For this review, take the finished solid that the model builds, in its own axes (mm). A direction names the side the tool comes from. Give positions to 0.01 mm unless a question says otherwise; leave off trailing zeros. Order: outer loops, then holes, each group sorted by start corner. A loop starts at its lowest first (then second) coordinate and runs counter-clockwise, first axis right, second up. Notation, with made-up numbers: (-20.5, 86.5) - (9.5, 86.5) arc R21 ccw to (9.5, 92.5) - close; hole circle Ø11 at (75, 26). An arc over 180 degrees is marked (long way). Put each result on its own line as item: value. Start each with the question number.
```python
from build123d import *

# Parameters (mm, degrees)
SKETCH1_W           = 69.43077851
SKETCH1_H           = 69.43077851
BOSS_EXTRUDE2_DEPTH = 3
SKETCH6_R           = 1.5
SKETCH6_W           = 50.43077851
SKETCH6_H           = 15.826208999
CUT_EXTRUDE1_DEPTH  = 10
FILLET1_R           = 10
FILLET2_R           = 10
FILLET3_R           = 4.994579941


with BuildPart() as part:
    # Sketch1 → Boss-Extrude2 (new body)
    with BuildSketch(Plane.XY):
        Rectangle(SKETCH1_W, SKETCH1_H)
    extrude(amount=BOSS_EXTRUDE2_DEPTH)

    # Sketch6 → Cut-Extrude1 (cut)
    with BuildSketch(Plane.XY.offset(3)):
        with Locations((-29, 24.5)):
            Circle(SKETCH6_R)
        with Locations((-29, -24.5)):
            Circle(SKETCH6_R)
        with Locations((29, -24.5)):
            Circle(SKETCH6_R)
        with Locations((29, 24.5)):
            Circle(SKETCH6_R)
        with Locations((0, -26.802284756)):
            Rectangle(SKETCH6_W, SKETCH6_H)
    extrude(amount=-CUT_EXTRUDE1_DEPTH, mode=Mode.SUBTRACT)

    # Fillet1
    fillet1_edges = [part.edges().sort_by_distance(p)[0] for p in [
        (34.715389255, 34.715389255, 1.5),
    ]]
    fillet(fillet1_edges, radius=FILLET1_R)

    # Fillet2
    # the kernel refuses this fillet: 10 mm, written as the material it takes off along each edge
    with BuildSketch(Plane(origin=(34.715389255, -34.715389255, -24.968730444), x_dir=(0, 1, 0), z_dir=(0, 0, 1))) as fillet2_piece_1:
        with BuildLine():
            CenterArc((9.987492178, 10), FILLET2_R, 182.865983983, 87.134016017)
            Line((0, 9.5), (-0.199749844, 9.49))
            ThreePointArc((-0.199749844, 9.49), (-0.2, 4.75), (-0.2, 0))
            Line((-0.2, 0), (0, -0.2))
            Line((0, -0.2), (9.987492178, -0.2))
            Line((9.987492178, -0.2), (9.987492178, 0))
        make_face()
    extrude(amount=52.937460889, mode=Mode.SUBTRACT)
    with BuildSketch(Plane(origin=(-34.715389255, -34.715389255, -24.968730444), x_dir=(0, 1, 0), z_dir=(0, 0, 1))) as fillet2_piece_2:
        with BuildLine():
            CenterArc((9.987492178, -10), FILLET2_R, 90, 87.134016017)
            Line((0, -9.5), (-0.199749844, -9.49))
            ThreePointArc((-0.199749844, -9.49), (-0.2, -4.75), (-0.2, 0))
            Line((-0.2, 0), (0, 0.2))
            Line((0, 0.2), (9.987492178, 0.2))
            Line((9.987492178, 0.2), (9.987492178, 0))
        make_face()
    extrude(amount=52.937460889, mode=Mode.SUBTRACT)
    with BuildSketch(Plane(origin=(-34.715389255, 34.715389255, -25), x_dir=(1, 0, 0), z_dir=(0, 0, 1))) as fillet2_piece_3:
        with BuildLine():
            CenterArc((FILLET2_R, -FILLET2_R), FILLET2_R, 90, 90)
            Line((0, -FILLET2_R), (-FILLET2_R * 0.02, -FILLET2_R))
            Line((-FILLET2_R * 0.02, -FILLET2_R), (-FILLET2_R * 0.02, FILLET2_R * 0.02))
            Line((-FILLET2_R * 0.02, FILLET2_R * 0.02), (FILLET2_R, FILLET2_R * 0.02))
            Line((FILLET2_R, FILLET2_R * 0.02), (FILLET2_R, 0))
        make_face()
    extrude(amount=53, mode=Mode.SUBTRACT)

    # Fillet3
    fillet3_edges = [part.edges().sort_by_distance(p)[0] for p in [
        (-25.215389255, -18.889180256, 1.5),
        (25.215389255, -18.889180256, 1.5),
    ]]
    fillet(fillet3_edges, radius=FILLET3_R)


solid = part.part
```
1. Add section C-C, the plane x = -29. Give the boundary of the cut face in (y, z), then the cut area to 3 significant figures.
2. Tool access review of faces 1 (the face through (25.215, -29, 2)), 2 (the face through (31.887, -31.697, 1.479)): name each direction out of +Z, -Z, +X, -X, +Y, -Y from which nothing blocks a thin tool from reaching the whole face with its end or side.
3. Add section D-D, the plane x = 23. Give the boundary of the cut face in (y, z), then the cut area to 3 significant figures.
4. The part is to be moulded in two halves that separate along Y. For faces 3 (the face through (0, 34.715, 1)), 4 (the face through (-32.034, -31.542, 1.479)), 5 (the face through (-30.11, -23.49, 1.52)), 6 (the face through (27.89, -23.49, 1.52)), say which applies: released by +Y, released by -Y, zero draft, split by the parting line, or undercut.
5. Clearance check with flat-ended pins moving along their axes: pin 1 (1.5 mm diameter, centred on y = -29.5, z = 1.5, fed in from +X); pin 2 (0.9 mm diameter, centred on x = 6.5, z = 1, fed in from -Y); pin 3 (1.5 mm diameter, centred on y = -31, z = 1, fed in from -X). State where each tip first meets the part, or that it passes through.
6. Add section A-A, the plane z = 2. Give the boundary of the cut face in (x, y), then the cut area to 3 significant figures.
7. Wall thickness on line 1 (Y direction, x = -30, z = 0.65); line 2 (Y direction, x = -28.5, z = 2.75); line 3 (X direction, y = -28, z = 0.55): over which ranges is each line inside the solid? List them lowest first. Write a range as from..to.
8. Add section B-B, the plane y = -20. Give the boundary of the cut face in (x, z).
Found:
1. outline: (-33.76, 0) - (-26, 0) - (-26, 3) - (-33.76, 3) - close; (-23, 0) - (23, 0) - (23, 3) - (-23, 3) - close; (26, 0) - (33.75, 0) - (33.75, 3) - (26, 3) - close
1. area: 185 mm^2
2. face 1: +Z, -Z, -Y
2. face 2: +Z, -Z, +X, -Y
3. outline: (-19.73, 0) - (34.72, 0) - (34.72, 3) - (-19.73, 3) - close
3. area: 163 mm^2
4. face 3: released by +Y
4. face 4: released by -Y
4. face 5: undercut
4. face 6: undercut
5. pin 1: stops at x = 33.87
5. pin 2: stops at y = -18.89
5. pin 3: stops at x = -33.05
6. outline: (-34.72, -24.73) arc R10 ccw to (-25.22, -34.72) - (-25.22, -23.88) arc R4.99 cw to (-20.22, -18.89) - (20.22, -18.89) arc R4.99 cw to (25.22, -23.88) - (25.22, -34.72) arc R10 ccw to (34.72, -24.73) - (34.72, 24.72) arc R10 ccw to (24.72, 34.72) - (-24.72, 34.72) arc R10 ccw to (-34.72, 24.72) - close; hole circle Ø3 at (-29, -24.5); hole circle Ø3 at (-29, 24.5); hole circle Ø3 at (29, -24.5); hole circle Ø3 at (29, 24.5)
6. area: 3,920 mm^2
7. line 1: y = -33.22..-25.62, -23.38..23.38, 25.62..33.2
7. line 2: y = -33.98..-25.91, -23.09..23.09, 25.91..33.97
7. line 3: x = -34.16..-25.22, 25.22..34.16
8. outline: (-34.72, 0) - (-23.36, 0) - (-23.36, 3) - (-34.72, 3) - close; (23.36, 0) - (34.72, 0) - (34.72, 3) - (23.36, 3) - close
